from build123d import *

# Parameters (mm, degrees)
SKETCH1_W           = 40
SKETCH1_H           = 13
BOSS_EXTRUDE1_DEPTH = 3
SKETCH3_R           = 1.25
CUT_EXTRUDE2_DEPTH  = 22.242645786
CUT_EXTRUDE3_DEPTH  = 10
FILLET2_R           = 5
FILLET3_R           = 1
FILLET4_R           = 5
FILLET5_R           = 5
SKETCH6_W           = 15.217676948
SKETCH6_H           = 27.138085695
CUT_EXTRUDE5_DEPTH  = 10


with BuildPart() as part:
    # Sketch1 → Boss-Extrude1 (new body)
    with BuildSketch(Plane(origin=(0, 0, 0), x_dir=(1, 0, 0), z_dir=(0, 1, 0))):
        Rectangle(SKETCH1_W, SKETCH1_H)
    extrude(amount=BOSS_EXTRUDE1_DEPTH)

    # Sketch3 → Cut-Extrude2 (cut, through all)
    with BuildSketch(Plane(origin=(0, 3, 0), x_dir=(1, 0, 0), z_dir=(0, 1, 0))):
        with Locations(Location((-17, 4, 0), (0, 0, 270))):
            Circle(SKETCH3_R)
        with Locations(Location((-17, -4, 0), (0, 0, 270))):
            Circle(SKETCH3_R)
    extrude(amount=-CUT_EXTRUDE2_DEPTH, mode=Mode.SUBTRACT)

    # Sketch5 → Cut-Extrude3 (cut)
    with BuildSketch(Plane(origin=(0, 3, 0), x_dir=(1, 0, 0), z_dir=(0, 1, 0))):
        with BuildLine():
            Line((-13.458222524, 6.5), (20, 0))
            Line((20, 0), (20, -6.5))
            Line((20, -6.5), (17.030073052, -6.5))
            ThreePointArc((17.030073052, -6.5), (7.775356774, -3.039372162), (-1.977274399, -4.624270773))
            Line((-1.977274399, -4.624270773), (-6.569653649, -6.5))
            Line((-6.569653649, -6.5), (-13.458222524, -6.5))
            Line((-13.458222524, -6.5), (-13.458222524, -10.237178745))
            Line((-13.458222524, -10.237178745), (26.023482417, -9.726914384))
            Line((26.023482417, -9.726914384), (26.023482417, 8.477274399))
            Line((26.023482417, 8.477274399), (-13.458222524, 8.477274399))
            Line((-13.458222524, 8.477274399), (-13.458222524, 6.5))
        make_face()
    extrude(amount=-CUT_EXTRUDE3_DEPTH, mode=Mode.SUBTRACT)

    # Fillet2
    fillet2_edges = [part.edges().sort_by_distance(p)[0] for p in [
        (-6.569653649, 1.5, 6.5),
        (-1.977274399, 1.5, 4.624270773),
        (17.030073052, 1.5, 6.5),
    ]]
    fillet(fillet2_edges, radius=FILLET2_R)

    # Fillet3
    fillet3_edges = [part.edges().sort_by_distance(p)[0] for p in [
        (20, 1.5, 6.5),
    ]]
    fillet(fillet3_edges, radius=FILLET3_R)

    # Fillet4
    fillet4_edges = [part.edges().sort_by_distance(p)[0] for p in [
        (20, 1.5, 0),
    ]]
    fillet(fillet4_edges, radius=FILLET4_R)

    # Fillet5
    fillet5_edges = [part.edges().sort_by_distance(p)[0] for p in [
        (-13.458222524, 1.5, -6.5),
    ]]
    fillet(fillet5_edges, radius=FILLET5_R)

    # Sketch6 → Cut-Extrude5 (cut)
    with BuildSketch(Plane(origin=(0, 3, 0), x_dir=(1, 0, 0), z_dir=(0, 1, 0))):
        with Locations((-17.629495701, -0.689660295)):
            Rectangle(SKETCH6_W, SKETCH6_H)
    extrude(amount=-CUT_EXTRUDE5_DEPTH, mode=Mode.SUBTRACT)


solid = part.part
Could you check a few things on this model? Use its own coordinates, in mm. A direction names the side the tool comes from. Give positions to 0.01 mm unless a question says otherwise; leave off trailing zeros. Order: outer loops, then holes, each group sorted by start corner. A loop starts at its lowest first (then second) coordinate and runs counter-clockwise, first axis right, second up.
1. For faces 4 (the flat face through (-9, 1, 6.5)), 5 (the cylindrical face through (-6.575, 1.479, 6.404)), which set-ups out of +Z, -Z, +X, -X, +Y, -Y let a thin tool reach every point of the face, with its end or its side?
2. We'd pull the mould along X, two halves only. Please class faces 1 (the flat face through (-3.793, 1.521, 5.366)), 2 (the flat face through (-10.021, 2, 0)), 3 (the flat face through (1, 0, 0)): pulls with the +X half, pulls with the -X half, needs draft (parallel to the pull), parting line crosses it, or undercut.
3. I need wall thicknesses on L1, parallel to X at y = 1.4, z = 6; L2, parallel to Z at x = 6, y = 0.3; L3, parallel to X at y = 1.5, z = 1. Which ranges of each line are inside material? Lowest first, please.
4. Suppose I cut it at D-D (z = -2). List the corners of the cut face in (x, y) for me, plus the area to 3 significant figures.
5. Suppose I cut it at A-A (y = 2.45). List the corners of the cut face in (x, z) for me, plus the area to 3 significant figures.
6. Suppose I cut it at B-B (z = 5). List the corners of the cut face in (x, y) for me, plus the area to 3 significant figures.
7. Suppose I cut it at C-C (x = -3.5). List the corners of the cut face in (y, z) for me, plus the area to 3 significant figures.
Solved:
1. face 4: +Z, +X, -X, +Y, -Y
1. face 5: +Z, +Y, -Y
2. face 1: undercut
2. face 2: pulls with the -X half
2. face 3: needs draft
3. L1: x = -10.02 to -5.35, 16.34 to 19.87
3. L2: z = -2.72 to 2.95
3. L3: x = -10.02 to 18.91
4. outline: (-10.02, 0) - (9.71, 0) - (9.71, 3) - (-10.02, 3) - close
4. area: 59.2 mm2
5. outline: (-10.02, -5.83) - (15.95, -0.79) arc R5 ccw to (20, 4.12) - (20, 5.5) arc R1 ccw to (19, 6.5) - (18.52, 6.5) arc R5 ccw to (15.92, 5.77) arc R19.26 cw to (-1.98, 4.62) - (-5.66, 6.13) arc R5 ccw to (-7.55, 6.5) - (-10.02, 6.5) - close
5. area: 224 mm2
6. outline: (-10.02, 0) - (-2.9, 0) - (-2.9, 3) - (-10.02, 3) - close; (14.54, 0) - (20, 0) - (20, 3) - (14.54, 3) - close
6. area: 37.8 mm2
7. outline: (0, -4.57) - (3, -4.57) - (3, 5.25) - (0, 5.25) - close
7. area: 29.4 mm2
